CAD build for the part. Positions are in the model's coordinates, mm. Face numbers are marked on the shaded views. Give positions to 0.01 mm unless a question says otherwise; leave off trailing zeros. Order: outer loops, then holes, each group sorted by start corner. A loop starts at its lowest first (then second) coordinate and runs counter-clockwise, first axis right, second up. Notation, with made-up numbers: (-12, 13.25) -> (-1, 13.25) arc R8 ccw to (-1, 19.25) -> close; hole circle Ø4 at (15.25, 39.5). An arc over 180 degrees is marked (long way). Answer as CSV lines item,"result".
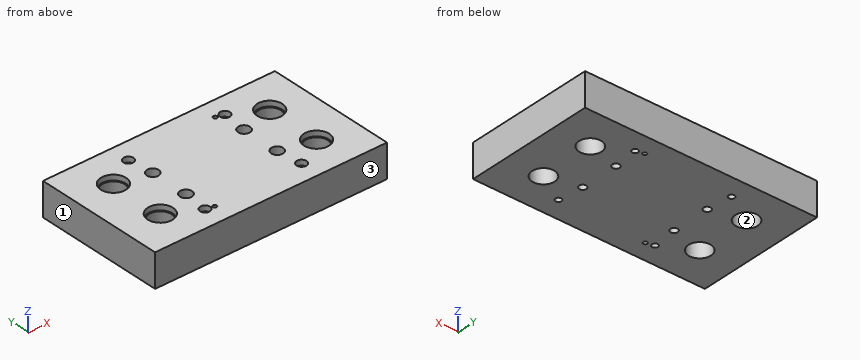
```python
from build123d import *

# Parameters (mm, degrees)
SKETCH1_W                       = 349.5
SKETCH1_H                       = 196
BOSS_EXTRUDE1_DEPTH             = 50
CBORE_FOR_M8_SHCS1_D            = 9
CBORE_FOR_M8_SHCS1_CBORE_D      = 15
CBORE_FOR_M8_SHCS1_CBORE_DEPTH  = 8
F_6_0MM_CLEARANCE_DOWEL_HOLE1_D = 6
CBORE_FOR_M10_SHSS1_D           = 11
CBORE_FOR_M10_SHSS1_CBORE_D     = 18
CBORE_FOR_M10_SHSS1_CBORE_DEPTH = 14.5
HOLE1_D                         = 34
HOLE1_CBORE_D                   = 38
HOLE1_CBORE_DEPTH               = 8


with BuildPart() as part:
    # Sketch1 → Boss-Extrude1 (new body)
    with BuildSketch(Plane.XY):
        with Locations((34.75, 0)):
            Rectangle(SKETCH1_W, SKETCH1_H)
    extrude(amount=BOSS_EXTRUDE1_DEPTH)

    # CBORE for M8 SHCS1 (through all)
    with Locations(Plane(origin=(0, 0, 50), x_dir=(0.9063077870366375, -0.42261826174072625, 0), z_dir=(0, 0, 1))):
        with Locations((125.743510643, -15.291158594), (69.11266357, 106.154084869), (-62.755119444, 44.663127785), (-6.124272371, -76.782115678)):
            CounterBoreHole(CBORE_FOR_M8_SHCS1_D / 2, CBORE_FOR_M8_SHCS1_CBORE_D / 2, CBORE_FOR_M8_SHCS1_CBORE_DEPTH)

    # Ø6.0mm Clearance Dowel Hole1 (through all)
    with Locations(Plane(origin=(0, 0, 50), x_dir=(0.9063077870366375, -0.42261826174072625, 0), z_dir=(0, 0, 1))):
        with Locations((56.96911534, 103.801589089), (6.019275859, -74.429619898)):
            Hole(F_6_0MM_CLEARANCE_DOWEL_HOLE1_D / 2)

    # CBORE for M10 SHSS1 (through all)
    with Locations(Plane(origin=(0, 0, 50), x_dir=(0.9063077870366375, -0.42261826174072625, 0), z_dir=(0, 0, 1))):
        with Locations((-43.07039435, 11.913904925), (-18.558535169, -40.651946723), (81.546926368, 70.023915914), (106.058785549, 17.458064266)):
            CounterBoreHole(CBORE_FOR_M10_SHSS1_D / 2, CBORE_FOR_M10_SHSS1_CBORE_D / 2, CBORE_FOR_M10_SHSS1_CBORE_DEPTH)

    # Hole1 (through all)
    with Locations(Plane(origin=(-83, 41, 50), x_dir=(1, 0, 0), z_dir=(0, 0, 1))):
        with Locations((0, 0), (0, -82), (235.5, 0), (235.5, -82)):
            CounterBoreHole(HOLE1_D / 2, HOLE1_CBORE_D / 2, HOLE1_CBORE_DEPTH)


solid = part.part
```
1) Band-saw the part on A-A, the plane x = 152.5. Write the cut outline in (y, z).
Data:
outline,"(-98, 0) -> (-58, 0) -> (-58, 42) -> (-60, 42) -> (-60, 50) -> (-98, 50) -> close; (-24, 0) -> (24, 0) -> (24, 42) -> (22, 42) -> (22, 50) -> (-22, 50) -> (-22, 42) -> (-24, 42) -> close; (58, 0) -> (98, 0) -> (98, 50) -> (60, 50) -> (60, 42) -> (58, 42) -> close"
2) Wall check: line 1 along Y through (x, z) = (-83, 26); line 2 along X through (y, z) = (40, 15); line 3 along Y through (x, z) = (-38, 47). Give the ranges that are in metal, low to high. Write a range as [from, to].
Data:
line 1,"y = [-98, -58], [-24, 24], [58, 98]"
line 2,"x = [-140, -99.97], [-66.03, 135.53], [169.47, 209.5]"
line 3,"y = [-98, -74.5], [-59.5, -37.06], [-20.94, 20.94], [37.06, 59.5], [74.5, 98]"
3) Band-saw the part on C-C, the plane x = -74. Write the cut outline in (y, z).
Data:
outline,"(-98, 0) -> (-55.42, 0) -> (-55.42, 42) -> (-57.73, 42) -> (-57.73, 50) -> (-98, 50) -> close; (-26.58, 0) -> (26.58, 0) -> (26.58, 42) -> (24.27, 42) -> (24.27, 50) -> (-24.27, 50) -> (-24.27, 42) -> (-26.58, 42) -> close; (55.42, 0) -> (98, 0) -> (98, 50) -> (57.73, 50) -> (57.73, 42) -> (55.42, 42) -> close"
4) Pin check, flat tip, straight feed: P1, Ø12, axis at x = -38, y = -67, coming from the +Z side. Stop position of the tip, or through.
Data:
P1,"stops at z = 42"
5) Band-saw the part on B-B, the plane z = 28.5. Give the number of separate pieces and of enclosed holes in the cut face, then the cut area to 3 significant figures.
Data:
separate pieces,"1"
enclosed holes,"14"
area,"64,200 mm2"
6) Pull direction Y, two halves, no side cores. Call the marked faces 1, 2 and 3: pulls with the +Y half, pulls with the -Y half, needs draft (parallel to the pull), parting line crosses it, or undercut.
Data:
face 1,"needs draft"
face 2,"undercut"
face 3,"pulls with the -Y half"
